Can you work these out from the model? Positions are in its coordinate system, mm. A direction names the side the tool comes from. Coordinates: 2 decimals unless noted, no trailing zeros. Order: outer loops, then holes, each group sorted by start corner. A loop starts at its lowest first (then second) coordinate and runs counter-clockwise, first axis right, second up. Notation, with made-up numbers: (-26.5, 64) -> (-19.5, 64) arc R26 cw to (-19.5, 87) -> close; hole circle Ø5 at (63.25, 15.25). An arc over 180 degrees is marked (long way). Answer as CSV lines item,"result".
from build123d import *

# Parameters (mm, degrees)
BOSS_EXTRUDE1_DEPTH      = 3
SKETCH2_3_R              = 4.25
SKETCH2_3_R_2            = 3
BOSS_EXTRUDE2_DEPTH      = 6
BOSS_EXTRUDE3_DEPTH      = 6
BOSS_EXTRUDE3_DEPTH_BACK = 3
SKETCH2_4_R              = 4.25
SKETCH2_4_R_2            = 3


with BuildPart() as part:
    # Sketch2 → Boss-Extrude1 (new body)
    with BuildSketch(Plane(origin=(0, 0, 0), x_dir=(1, 0, 0), z_dir=(0, 1, 0))):
        with BuildLine():
            ThreePointArc((21, -2), (20.5, 0), (21, 2))
            Line((21, 2), (-21, 2))
            ThreePointArc((-21, 2), (-20.626894374, 1.030776406), (-20.5, 0))
            ThreePointArc((-20.5, 0), (-20.626894374, -1.030776406), (-21, -2))
            Line((-21, -2), (21, -2))
        make_face()
    extrude(amount=BOSS_EXTRUDE1_DEPTH)

    # Sketch2_3 → Boss-Extrude2 (add)
    with BuildSketch(Plane(origin=(0, 0, 0), x_dir=(1, 0, 0), z_dir=(0, 1, 0))):
        with Locations(Location((-24.75, 0, 0), (0, 0, 28.072486936))):
            Circle(SKETCH2_3_R)
        with Locations(Location((-24.75, 0, 0), (0, 0, 270))):
            Circle(SKETCH2_3_R_2, mode=Mode.SUBTRACT)
    extrude(amount=BOSS_EXTRUDE2_DEPTH)

    # Sketch2_4 → Boss-Extrude3 (add, two sides: drawn at the far end of the back side and taken through both)
    with BuildSketch(Plane(origin=(0, 0, 0), x_dir=(1, 0, 0), z_dir=(0, 1, 0)).offset(-BOSS_EXTRUDE3_DEPTH_BACK)):
        with Locations(Location((24.75, 0, 0), (0, 0, 270))):
            Circle(SKETCH2_4_R)
        with Locations(Location((24.75, 0, 0), (0, 0, 270))):
            Circle(SKETCH2_4_R_2, mode=Mode.SUBTRACT)
    extrude(amount=BOSS_EXTRUDE3_DEPTH + BOSS_EXTRUDE3_DEPTH_BACK)


solid = part.part
Q1. Imagine slicing it at D-D (y = 5). List the corners of the cut face in (x, z) for me, and give its area (3 significant figures).
Solution:
outline,"circle Ø8.5 at (-24.75, 0); circle Ø8.5 at (24.75, 0); hole circle Ø6 at (-24.75, 0); hole circle Ø6 at (24.75, 0)"
area,"56.9 mm2"
Q2. For P1, Ø4, axis at x = -17, z = -3, coming from the -Y side; P2, Ø4, axis at y = -2, z = -3, coming from the +X side; P3, Ø4, axis at y = 0, z = -2, coming from the -X side; P4, Ø0.9, axis at x = 7, y = 2, coming from the -Z side, each with a flat end and sliding along its axis, tell me the tip position at first contact or that it passes through.
Solution:
P1,"y = 0"
P2,"x = 28.88"
P3,"x = -29"
P4,"z = -2"
Q3. Imagine slicing it at C-C (y = 0.75). List the corners of the cut face in (x, z) for me.
Solution:
outline,"(-21, -2) -> (21, -2) arc R4.25 ccw (long way) to (21, 2) -> (-21, 2) arc R4.25 ccw (long way) to start; hole circle Ø6 at (-24.75, 0); hole circle Ø6 at (24.75, 0)"
Q4. Imagine slicing it at A-A (z = 0). List the corners of the cut face in (x, y) for me, and give its area (4 significant figures).
Solution:
outline,"(-29, 0) -> (-27.75, 0) -> (-27.75, 6) -> (-29, 6) -> close; (-21.75, 0) -> (20.5, 0) -> (20.5, -3) -> (21.75, -3) -> (21.75, 6) -> (20.5, 6) -> (20.5, 3) -> (-20.5, 3) -> (-20.5, 6) -> (-21.75, 6) -> close; (27.75, -3) -> (29, -3) -> (29, 6) -> (27.75, 6) -> close"
area,"160.5 mm2"
Q5. Imagine slicing it at B-B (x = 24.75). List the corners of the cut face in (y, z) for me.
Solution:
outline,"(-3, -4.25) -> (6, -4.25) -> (6, -3) -> (-3, -3) -> close; (-3, 3) -> (6, 3) -> (6, 4.25) -> (-3, 4.25) -> close"
Q6. If I drill on line 1 (X direction, y = 3.7, z = 0); line 2 (X direction, y = 2.75, z = -0.25); line 3 (Z direction, x = -25, y = 0.25), over which ranges is the centre line in solid material (lowest first)?
Solution:
line 1,"-29 to -27.75, -21.75 to -20.5, 20.5 to 21.75, 27.75 to 29"
line 2,"-28.99 to -27.74, -21.76 to 21.76, 27.74 to 28.99"
line 3,"-4.24 to -2.99, 2.99 to 4.24"
Q7. Which directions (+Z, -Z, +X, -X, +Y, -Y) give clear straight access to the entire face, cutting with the end or side of a thin tool? Please do faces 1 (the flat face through (0, 1, 2)), 2 (the flat face through (-28, 6, 0)).
Solution:
face 1,"+Z, +Y, -Y"
face 2,"+Z, -Z, +X, -X, +Y"
Q8. We'd pull the mould along Z, two halves only. Please class faces 3 (the cylindrical face through (-28.866, 2.958, -1.06)), 4 (the cylindrical face through (25.65, 1.44, 2.86)), 5 (the flat face through (0, 1, -2)): pulls with the +Z half, pulls with the -Z half, needs draft (parallel to the pull), parting line crosses it, or undercut.
Solution:
face 3,"parting line crosses it"
face 4,"undercut"
face 5,"pulls with the -Z half"
